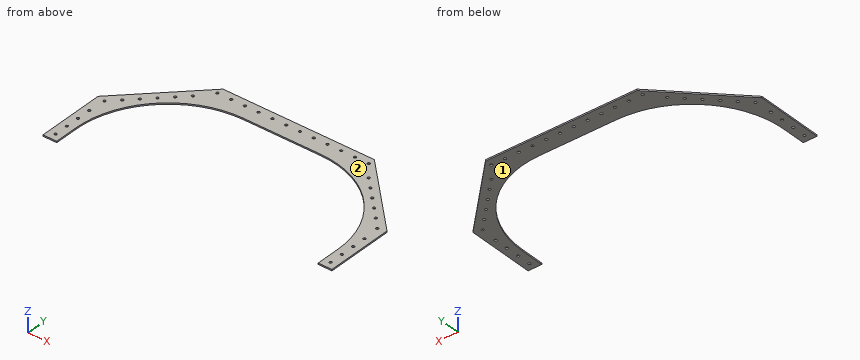
```python
from build123d import *

# Parameters (mm, degrees)
BOSS_EXTRUDE1_DEPTH   = 2.54
F_8_CLEARANCE_HOLE1_D = 4.9149


with BuildPart() as part:
    # Sketch1 → Boss-Extrude1 (new body)
    with BuildSketch(Plane.XY):
        with BuildLine():
            Line((266.7, 0), (241.3, 0))
            Line((241.3, 0), (241.3, 43.70119491))
            ThreePointArc((241.3, 43.70119491), (191.589487758, 163.712987758), (71.57769491, 213.4235))
            Line((71.57769491, 213.4235), (-71.57769491, 213.4235))
            ThreePointArc((-71.57769491, 213.4235), (-191.589487758, 163.712987758), (-241.3, 43.70119491))
            Line((-241.3, 43.70119491), (-241.3, 0))
            Line((-241.3, 0), (-266.7, 0))
            Line((-266.7, 0), (-266.7, 124.5235))
            Line((-266.7, 124.5235), (-139.7, 251.5235))
            Line((-139.7, 251.5235), (139.7, 251.5235))
            Line((139.7, 251.5235), (266.7, 124.5235))
            Line((266.7, 124.5235), (266.7, 0))
        make_face()
    extrude(amount=BOSS_EXTRUDE1_DEPTH)

    # #8 Clearance Hole1 (through all)
    with Locations(Plane(origin=(0, 0, 0), x_dir=(-1, 0, 0), z_dir=(0, 0, -1))):
        with Locations((-254, 12.7635), (-254, 38.1635), (-254, 63.5635), (-254, 88.9635), (-251.804819447, 120.777889402), (-234.083674396, 139.179313362), (-216.123162153, 157.139825604), (-198.162649911, 175.100337847), (-180.202137669, 193.060850089), (-162.241625427, 211.021362331), (-114.3, 238.8235), (-88.9, 238.8235), (-63.5, 238.8235), (-38.1, 238.8235), (-12.7, 238.8235), (12.7, 238.8235), (38.1, 238.8235), (63.5, 238.8235), (88.9, 238.8235), (114.3, 238.8235), (139.7, 238.8235), (162.241625427, 211.021362331), (180.202137669, 193.060850089), (198.162649911, 175.100337847), (216.123162153, 157.139825604), (234.083674396, 139.179313362), (252.044186638, 121.21880112), (254, 88.9635), (254, 63.5635), (254, 38.1635), (254, 12.7635), (-139.7, 238.8235)):
            Hole(F_8_CLEARANCE_HOLE1_D / 2)


solid = part.part
```
Here's how the part is built. I have some questions about the finished solid (model axes, mm). Face numbers are marked on the shaded views. Give positions to 0.01 mm unless a question says otherwise; leave off trailing zeros. Loops run counter-clockwise (first coordinate to the right, second up) from the corner with the lowest first, then second, coordinate; pieces in that order, holes last. Notation, with made-up numbers: M -32.5,55 L 2.5,55 A14 ccw 2.5,72 Z; hole C -3.5,19.5 d2. An arc over 180 degrees is marked long. Use one line per item in the form item = value. Start each with the question number.
Q1. Thinking about a two-plate mould opening in Z: for the marked faces 1 and 2, which applies, +Z half, -Z half, draft (parallel to the pull), parting line (faces both ways), or undercut?
Q2. If we section it at A-A (x = 49.5): Write out the boundary of the cut face in (y, z), then the cut area to 3 significant figures.
Q3. If we section it at C-C (x = -149.5): Write out the boundary of the cut face in (y, z), then the cut area to 3 significant figures.
Q4. I need wall thicknesses on line 1 along Y through (x, z) = (-63.5, 0.8); line 2 along X through (y, z) = (62.5, 2.35); line 3 along X through (y, z) = (192.5, 1.3). Which ranges of each line are inside material? Lowest first, please.
Q5. If we section it at B-B (z = 0.7): State how many separate pieces and enclosed holes the cut face has, then the cut area to 3 significant figures.
Q6. Will this pin go through, and if not, where does the flat tip stop? pin 1 Ø0.8 at (x, z) = (31.5, 1.5) entering from -Y.
Taken from the geometry:
q1.face_1 = -Z half
q1.face_2 = +Z half
q2.outline = M 213.42,0 L 251.52,0 L 251.52,2.54 L 213.42,2.54 Z
q2.area = 96.8 mm^2
q3.outline = M 194.48,0 L 241.72,0 L 241.72,2.54 L 194.48,2.54 Z
q3.area = 120 mm^2
q4.line_1 = 213.42 to 236.37, 241.28 to 251.52
q4.line_2 = -266.7 to -256.22, -251.78 to -240.26, 240.26 to 251.78, 256.22 to 266.7
q4.line_3 = -198.72 to -182.59, -177.81 to -153.21, 153.21 to 177.81, 182.59 to 198.72
q5.separate_pieces = 1
q5.enclosed_holes = 32
q5.area = 26,800 mm^2
q6.pin_1 = 213.42
